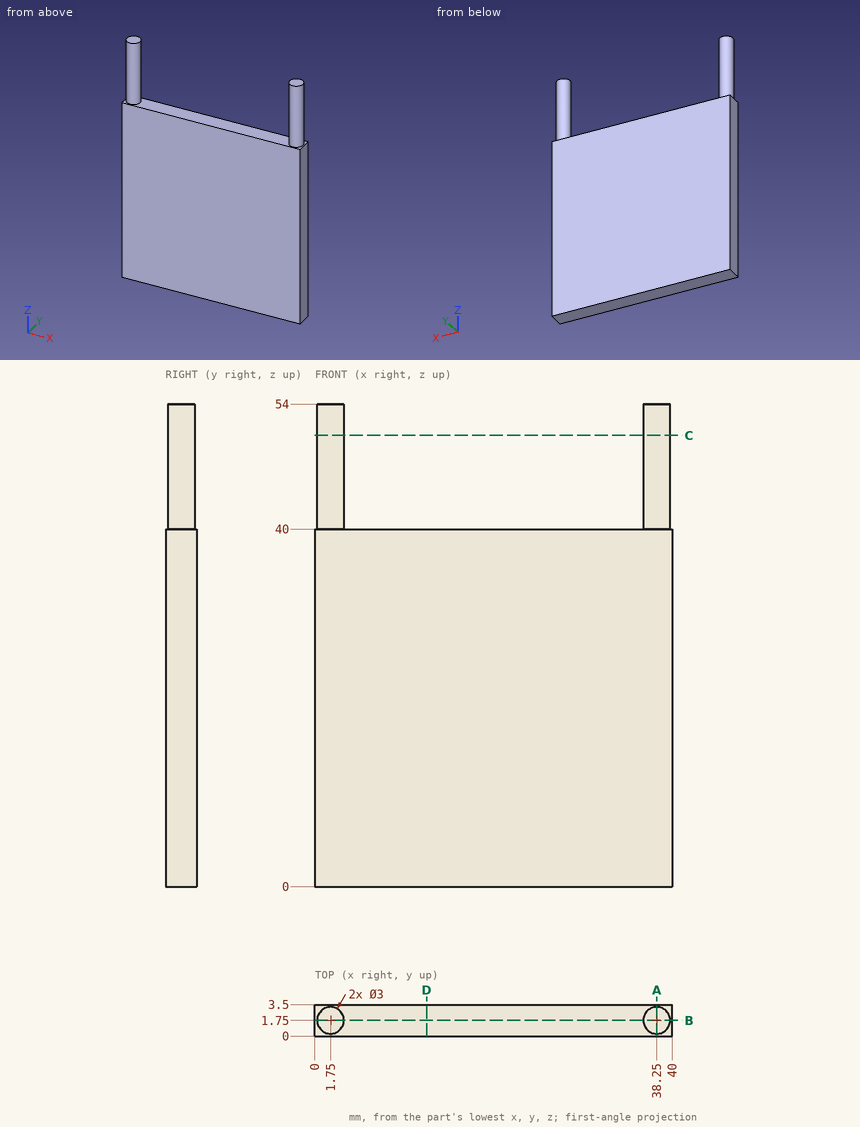
Here's the drawing with two shaded views (mm, measured from the low corner). I have some questions. Round coordinates to 2 decimals unless told otherwise and drop trailing zeros. Write each loop counter-clockwise with the first axis right and the second up, starting at its lowest first coordinate (ties: lowest second). Pieces come first, ordered by that corner, then holes.
(1) Suppose I cut it at D-D on x = 12.5. Write out the boundary of the cut face in (y, z), and give its area (3 significant figures).
Findings below:
outline: (0, 0) - (3.5, 0) - (3.5, 40) - (0, 40) - close
area: 140 mm2
(2) For pin 1 (1 mm diameter, centred on x = 23.5, y = 2, fed in from +Z), with a flat end and sliding along its axis, tell me the tip position at first contact or that it passes through.
Findings below:
pin 1: stops at z = 40
(3) Suppose I cut it at C-C on z = 50.5. Write out the boundary of the cut face in (x, y).
Findings below:
outline: circle Ø3 at (1.75, 1.75); circle Ø3 at (38.25, 1.75)
(4) Suppose I cut it at B-B on y = 1.75. Write out the boundary of the cut face in (x, z), and give its area (3 significant figures).
Findings below:
outline: (0, 0) - (40, 0) - (40, 40) - (39.75, 40) - (39.75, 54) - (36.75, 54) - (36.75, 40) - (3.25, 40) - (3.25, 54) - (0.25, 54) - (0.25, 40) - (0, 40) - close
area: 1,680 mm2
(5) If I drill on probe 1 along Z at (x, y) = (23.5, 3.35), over which ranges is the centre line in solid material (lowest first)?
Findings below:
probe 1: z = 0 to 40
(6) Suppose I cut it at A-A on x = 38.25. Write out the boundary of the cut face in (y, z).
Findings below:
outline: (0, 0) - (3.5, 0) - (3.5, 40) - (3.25, 40) - (3.25, 54) - (0.25, 54) - (0.25, 40) - (0, 40) - close
